```python
from build123d import *

# Parameters (mm, degrees)
F0_W     = 147
F0_H     = 206
F0_W_2   = 2
F0_H_2   = 1
F0_W_3   = 1
F1_DEPTH = 2
F2_DEPTH = 4


with BuildPart() as f1:
    # F0 (on Top) → F1 (new body)
    with BuildSketch(Plane.XY):
        with Locations((0, -2)):
            Rectangle(F0_W, F0_H)
        Polygon((77.5, 102), (77.5, 104), (76.5, 104), (74.5, 104), (73.5, 104), (-73.5, 104), (-74.5, 104), (-76.5, 104), (-77.5, 104), (-77.5, 102), (-76.5, 102), (-74.5, 102), (-73.5, 102), (73.5, 102), (74.5, 102), (76.5, 102), align=None)
        with Locations((75.5, -2)):
            Rectangle(F0_W_2, F0_H)
        with Locations((-75.5, -2)):
            Rectangle(F0_W_2, F0_H)
        with Locations((0, 101.5)):
            Rectangle(F0_W, F0_H_2)
        with Locations((74, -2)):
            Rectangle(F0_W_3, F0_H)
        with Locations((-74, -2)):
            Rectangle(F0_W_3, F0_H)
        with Locations((0, 104.5)):
            Rectangle(F0_W, F0_H_2)
        with Locations((-77, -2)):
            Rectangle(F0_W_3, F0_H)
        with Locations((77, -2)):
            Rectangle(F0_W_3, F0_H)
        with Locations((-74, 101.5)):
            Rectangle(F0_W_3, F0_H_2)
        with Locations((75.5, 101.5)):
            Rectangle(F0_W_2, F0_H_2)
        with Locations((74, 101.5)):
            Rectangle(F0_W_3, F0_H_2)
        with Locations((77, 101.5)):
            Rectangle(F0_W_3, F0_H_2)
        with Locations((-77, 101.5)):
            Rectangle(F0_W_3, F0_H_2)
        with Locations((-74, 104.5)):
            Rectangle(F0_W_3, F0_H_2)
        with Locations((74, 104.5)):
            Rectangle(F0_W_3, F0_H_2)
        with Locations((-75.5, 101.5)):
            Rectangle(F0_W_2, F0_H_2)
        with Locations((-75.5, 104.5)):
            Rectangle(F0_W_2, F0_H_2)
        with Locations((-77, 104.5)):
            Rectangle(F0_W_3, F0_H_2)
        with Locations((77, 104.5)):
            Rectangle(F0_W_3, F0_H_2)
        with Locations((75.5, 104.5)):
            Rectangle(F0_W_2, F0_H_2)
    extrude(amount=F1_DEPTH)

    # F0 (on Top) → F2 (join)
    with BuildSketch(Plane.XY):
        with Locations((77, -2)):
            Rectangle(F0_W_3, F0_H)
        with Locations((77, 101.5)):
            Rectangle(F0_W_3, F0_H_2)
        with Locations((-77, -2)):
            Rectangle(F0_W_3, F0_H)
        with Locations((-77, 101.5)):
            Rectangle(F0_W_3, F0_H_2)
        with Locations((-74, 104.5)):
            Rectangle(F0_W_3, F0_H_2)
        with Locations((74, 104.5)):
            Rectangle(F0_W_3, F0_H_2)
        with Locations((0, 104.5)):
            Rectangle(F0_W, F0_H_2)
        with Locations((0, 101.5)):
            Rectangle(F0_W, F0_H_2)
        with Locations((-74, -2)):
            Rectangle(F0_W_3, F0_H)
        with Locations((74, -2)):
            Rectangle(F0_W_3, F0_H)
        with Locations((-74, 101.5)):
            Rectangle(F0_W_3, F0_H_2)
        with Locations((74, 101.5)):
            Rectangle(F0_W_3, F0_H_2)
    extrude(amount=F2_DEPTH)


solid = f1.part
```
The model under review builds one solid part; all positions refer to its coordinate system, in mm. A direction names the side the tool comes from. Round coordinates to 2 decimals unless told otherwise and drop trailing zeros. Loops run counter-clockwise (first coordinate to the right, second up) from the corner with the lowest first, then second, coordinate; pieces in that order, holes last. Notation, with made-up numbers: M -22,-26 L 6,-26 A15 cw 6,-18 Z; hole C 39.25,-0.75 d10. An arc over 180 degrees is marked long. Write item = value, one per line.
Item 1: Take a section at A-A on z = 2.75. Write out the cut boundary in (x, y).
Return value:
outline = M -77.5,-105 L -76.5,-105 L -76.5,102 L -77.5,102 Z; M -74.5,-105 L -73.5,-105 L -73.5,101 L 73.5,101 L 73.5,-105 L 74.5,-105 L 74.5,102 L -74.5,102 Z; M -74.5,104 L 74.5,104 L 74.5,105 L -74.5,105 Z; M 76.5,-105 L 77.5,-105 L 77.5,102 L 76.5,102 Z
Item 2: Take a section at C-C on x = -32.5. Write out the cut boundary in (y, z).
Return value:
outline = M -105,0 L 105,0 L 105,4 L 104,4 L 104,2 L 102,2 L 102,4 L 101,4 L 101,2 L -105,2 Z
Item 3: Insertion check: P1, Ø1, axis at x = -10, z = 3, coming from the -Y side; P2, Ø0.5, axis at y = 104.5, z = 2.5, coming from the +X side; P3, Ø0.5, axis at y = 104.5, z = 3.5, coming from the -X side. Each pin has a flat end and moves straight along its axis. Give the tip position at first contact, or say it passes through.
Return value:
P1 = 101
P2 = 74.5
P3 = -74.5
Item 4: Take a section at B-B on y = -17. Write out the cut boundary in (x, z), then the cut area to 3 significant figures.
Return value:
outline = M -77.5,0 L 77.5,0 L 77.5,4 L 76.5,4 L 76.5,2 L 74.5,2 L 74.5,4 L 73.5,4 L 73.5,2 L -73.5,2 L -73.5,4 L -74.5,4 L -74.5,2 L -76.5,2 L -76.5,4 L -77.5,4 Z
area = 318 mm2
Item 5: Machinability: for faces 1 (the flat face through (-77.5, 1, 2)), 2 (the flat face through (-1, -1, 2)), which of the approach directions +Z, -Z, +X, -X, +Y, -Y give a long, thin tool a straight path to every point of the face, cutting with its end or side? Answer none if there is none.
Return value:
face_1 = +Z, -Z, -X, +Y, -Y
face_2 = +Z, -Y
Item 6: For line 1 (X direction, y = 61, z = 2.3); line 2 (Y direction, x = -44, z = 3.4); line 3 (Z direction, x = -26, y = 34), list the stretches that pass through material, from the lowest coordinate up. Write a range as [from, to].
Return value:
line_1 = [-77.5, -76.5], [-74.5, -73.5], [73.5, 74.5], [76.5, 77.5]
line_2 = [101, 102], [104, 105]
line_3 = [0, 2]
